Geometry check sheet. Reference: the model listing, model coordinates, mm. Face numbers are marked on the shaded views. A direction names the side the tool comes from. Round coordinates to 2 decimals unless told otherwise and drop trailing zeros.
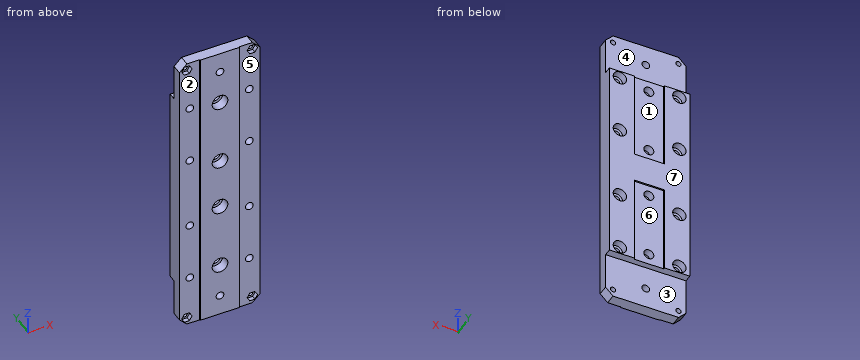
```python
from build123d import *

# Parameters (mm, degrees)
SKETCH1_W               = 54
SKETCH1_H               = 200
SKETCH1_R               = 2.6
SKETCH1_R_2             = 3.35
BOSS_EXTRUDE1_DEPTH     = 12
SKETCH4_R               = 5.25
CUT_EXTRUDE2_DEPTH      = 6
CUT_EXTRUDE3_START      = 12
SKETCH5_W               = 20
SKETCH5_H               = 60
CUT_EXTRUDE3_DEPTH      = 1
CUT_EXTRUDE4_DEPTH      = 105.273678366
CUT_EXTRUDE4_DEPTH_BACK = 105.273678366
SKETCH6_R               = 1.75
CUT_EXTRUDE5_DEPTH      = 3
CHAMFER2_SIZE           = 5
BOSS_EXTRUDE3_START     = -0.5
SKETCH9_W               = 27
SKETCH9_H               = 200
SKETCH9_R               = 2.6
SKETCH9_R_2             = 5.25
BOSS_EXTRUDE3_DEPTH     = 0.5
CHAMFER3_SIZE           = 0.5
SKETCH10_W              = 54
SKETCH10_H              = 30
CUT_EXTRUDE6_DEPTH      = 5
CUT_EXTRUDE7_START      = 12
SKETCH11_R              = 4.5
CUT_EXTRUDE7_DEPTH      = 5


with BuildPart() as part:
    # Sketch1 → Boss-Extrude1 (new body)
    with BuildSketch(Plane(origin=(0, 0, 0), x_dir=(1, 0, 0), z_dir=(0, 1, 0))):
        Rectangle(SKETCH1_W, SKETCH1_H)
        with Locations(Location((0, 86, 0), (0, 0, 270))):
            Circle(SKETCH1_R, mode=Mode.SUBTRACT)
        with Locations(Location((0, -86, 0), (0, 0, 270))):
            Circle(SKETCH1_R, mode=Mode.SUBTRACT)
        with Locations(Location((0, 62.5, 0), (0, 0, 270))):
            Circle(SKETCH1_R_2, mode=Mode.SUBTRACT)
        with Locations(Location((0, 17.5, 0), (0, 0, 270))):
            Circle(SKETCH1_R_2, mode=Mode.SUBTRACT)
        with Locations(Location((0, -17.5, 0), (0, 0, 270))):
            Circle(SKETCH1_R_2, mode=Mode.SUBTRACT)
        with Locations(Location((0, -62.5, 0), (0, 0, 270))):
            Circle(SKETCH1_R_2, mode=Mode.SUBTRACT)
        with Locations(Location((-20, -65, 0), (0, 0, 270))):
            Circle(SKETCH1_R, mode=Mode.SUBTRACT)
        with Locations(Location((20, -65, 0), (0, 0, 270))):
            Circle(SKETCH1_R, mode=Mode.SUBTRACT)
        with Locations(Location((20, -25, 0), (0, 0, 270))):
            Circle(SKETCH1_R, mode=Mode.SUBTRACT)
        with Locations(Location((-20, -25, 0), (0, 0, 270))):
            Circle(SKETCH1_R, mode=Mode.SUBTRACT)
        with Locations(Location((-20, 25, 0), (0, 0, 270))):
            Circle(SKETCH1_R, mode=Mode.SUBTRACT)
        with Locations(Location((20, 25, 0), (0, 0, 270))):
            Circle(SKETCH1_R, mode=Mode.SUBTRACT)
        with Locations(Location((20, 65, 0), (0, 0, 270))):
            Circle(SKETCH1_R, mode=Mode.SUBTRACT)
        with Locations(Location((-20, 65, 0), (0, 0, 270))):
            Circle(SKETCH1_R, mode=Mode.SUBTRACT)
    extrude(amount=BOSS_EXTRUDE1_DEPTH)

    # Sketch4 → Cut-Extrude2 (cut)
    with BuildSketch(Plane(origin=(0, 0, 0), x_dir=(1, 0, 0), z_dir=(0, 1, 0))):
        with Locations(Location((0, 62.5, 0), (0, 0, 270))):
            Circle(SKETCH4_R)
        with Locations(Location((0, 17.5, 0), (0, 0, 270))):
            Circle(SKETCH4_R)
        with Locations(Location((0, -17.5, 0), (0, 0, 270))):
            Circle(SKETCH4_R)
        with Locations(Location((0, -62.5, 0), (0, 0, 270))):
            Circle(SKETCH4_R)
    extrude(amount=CUT_EXTRUDE2_DEPTH, mode=Mode.SUBTRACT)

    # Sketch5 → Cut-Extrude3 (cut)
    with BuildSketch(Plane(origin=(0, 0, 0), x_dir=(1, 0, 0), z_dir=(0, 1, 0)).offset(CUT_EXTRUDE3_START)):
        with Locations((0, 40)):
            Rectangle(SKETCH5_W, SKETCH5_H)
        with Locations((0, -40)):
            Rectangle(SKETCH5_W, SKETCH5_H)
    extrude(amount=-CUT_EXTRUDE3_DEPTH, mode=Mode.SUBTRACT)

    # Sketch6 → Cut-Extrude4 (cut, two sides: drawn at the far end of the back side and taken through both)
    with BuildSketch(Plane(origin=(0, 0, 0), x_dir=(1, 0, 0), z_dir=(0, 1, 0)).offset(-CUT_EXTRUDE4_DEPTH_BACK)):
        with Locations(Location((22, 95, 0), (0, 0, 90))):
            Circle(SKETCH6_R)
        with Locations(Location((22, -95, 0), (0, 0, 90))):
            Circle(SKETCH6_R)
        with Locations(Location((-22, -95, 0), (0, 0, 90))):
            Circle(SKETCH6_R)
        with Locations(Location((-22, 95, 0), (0, 0, 90))):
            Circle(SKETCH6_R)
    extrude(amount=CUT_EXTRUDE4_DEPTH + CUT_EXTRUDE4_DEPTH_BACK, mode=Mode.SUBTRACT)

    # Sketch7 → Cut-Extrude5 (cut)
    with BuildSketch(Plane(origin=(0, 0, 0), x_dir=(1, 0, 0), z_dir=(0, 1, 0))):
        Polygon((18.535898385, 95), (20.267949192, 92), (23.732050808, 92), (25.464101615, 95), (23.732050808, 98), (20.267949192, 98), align=None)
        Polygon((18.535898385, -95), (20.267949192, -98), (23.732050808, -98), (25.464101615, -95), (23.732050808, -92), (20.267949192, -92), align=None)
        Polygon((-25.464101615, -95), (-23.732050808, -98), (-20.267949192, -98), (-18.535898385, -95), (-20.267949192, -92), (-23.732050808, -92), align=None)
        Polygon((-25.464101615, 95), (-23.732050808, 92), (-20.267949192, 92), (-18.535898385, 95), (-20.267949192, 98), (-23.732050808, 98), align=None)
    extrude(amount=CUT_EXTRUDE5_DEPTH, mode=Mode.SUBTRACT)

    # Chamfer2
    chamfer2_edges = [part.edges().sort_by_distance(p)[0] for p in [
        (27, 6, 100),
        (-27, 6, 100),
        (-27, 6, -100),
        (27, 6, -100),
    ]]
    chamfer(chamfer2_edges, length=CHAMFER2_SIZE)

    # Sketch9 → Boss-Extrude3 (add)
    with BuildSketch(Plane(origin=(0, 0, 0), x_dir=(1, 0, 0), z_dir=(0, 1, 0)).offset(BOSS_EXTRUDE3_START)):
        Rectangle(SKETCH9_W, SKETCH9_H)
        with Locations(Location((0, -86, 0), (0, 0, 270))):
            Circle(SKETCH9_R, mode=Mode.SUBTRACT)
        with Locations(Location((0, -62.5, 0), (0, 0, 270))):
            Circle(SKETCH9_R_2, mode=Mode.SUBTRACT)
        with Locations(Location((0, -17.5, 0), (0, 0, 270))):
            Circle(SKETCH9_R_2, mode=Mode.SUBTRACT)
        with Locations(Location((0, 17.5, 0), (0, 0, 270))):
            Circle(SKETCH9_R_2, mode=Mode.SUBTRACT)
        with Locations(Location((0, 62.5, 0), (0, 0, 270))):
            Circle(SKETCH9_R_2, mode=Mode.SUBTRACT)
        with Locations(Location((0, 86, 0), (0, 0, 270))):
            Circle(SKETCH9_R, mode=Mode.SUBTRACT)
    extrude(amount=BOSS_EXTRUDE3_DEPTH)

    # Chamfer3
    chamfer3_edges = [part.edges().sort_by_distance(p)[0] for p in [
        (-13.5, -0.5, 0),
        (13.5, -0.5, 0),
    ]]
    chamfer(chamfer3_edges, length=CHAMFER3_SIZE - 0.0001)  # a hair under: the kernel refuses the full size

    # Sketch10 → Cut-Extrude6 (cut)
    with BuildSketch(Plane(origin=(0, 12, 0), x_dir=(1, 0, 0), z_dir=(0, 1, 0))):
        with Locations((0, -85)):
            Rectangle(SKETCH10_W, SKETCH10_H)
        with Locations((0, 85)):
            Rectangle(SKETCH10_W, SKETCH10_H)
    extrude(amount=-CUT_EXTRUDE6_DEPTH, mode=Mode.SUBTRACT)

    # Sketch11 → Cut-Extrude7 (cut)
    with BuildSketch(Plane(origin=(0, 0, 0), x_dir=(1, 0, 0), z_dir=(0, 1, 0)).offset(CUT_EXTRUDE7_START)):
        with Locations(Location((20, 65, 0), (0, 0, 90))):
            Circle(SKETCH11_R)
        with Locations(Location((-20, 65, 0), (0, 0, 90))):
            Circle(SKETCH11_R)
        with Locations(Location((-20, 25, 0), (0, 0, 90))):
            Circle(SKETCH11_R)
        with Locations(Location((20, 25, 0), (0, 0, 90))):
            Circle(SKETCH11_R)
        with Locations(Location((20, -25, 0), (0, 0, 90))):
            Circle(SKETCH11_R)
        with Locations(Location((-20, -25, 0), (0, 0, 90))):
            Circle(SKETCH11_R)
        with Locations(Location((-20, -65, 0), (0, 0, 90))):
            Circle(SKETCH11_R)
        with Locations(Location((20, -65, 0), (0, 0, 90))):
            Circle(SKETCH11_R)
    extrude(amount=-CUT_EXTRUDE7_DEPTH, mode=Mode.SUBTRACT)


solid = part.part
```
1) Gauge pin test, flat ends, axial feed: pin 1 (4.5 mm diameter, centred on x = 22, z = 95, fed in from -Y); pin 2 (4 mm diameter, centred on x = -20, z = 65, fed in from +Y); pin 3 (1.5 mm diameter, centred on x = 5.5, y = 8.5, fed in from +Z); pin 4 (7 mm diameter, centred on x = -19, z = 24, fed in from +Y). Record the tip position at first contact, or that the pin passes through.
Report:
pin 1: stops at y = 3
pin 2: passes through
pin 3: stops at z = 70
pin 4: stops at y = 12
2) Sectioned sample at B-B, the plane z = 25. State how many separate pieces and enclosed holes the cut face has, then the cut area to 3 significant figures.
Report:
separate pieces: 3
enclosed holes: 0
area: 478 mm2
3) Mould release check, pull along X, two halves, no side actions. Record for the marked faces 1 and 2: +X half, -X half, draft (parallel to the pull), parting line (faces both ways), or undercut.
Report:
face 1: undercut
face 2: draft
4) Access from +Z, -Z, +X, -X, +Y, -Y to the whole of each face (thin tool, end or side, straight path). Record for the marked faces 3, 4, 5, 6 and 7.
Report:
face 3: -Z, +X, -X, +Y
face 4: +Z, +X, -X, +Y
face 5: +Z, -Z, +X, -Y
face 6: -Z, +Y
face 7: +Z, -Z, +X, -X, +Y
5) Scan lines: line 1 along Z through (x, y) = (0, 9); line 2 along X through (y, z) = (9.3, -25); line 3 along Z through (x, y) = (20, 5.75). Record each from-to range of solid material in increasing order.
Report:
line 1: z = -70 to -65.85, -59.15 to -20.85, -14.15 to 14.15, 20.85 to 59.15, 65.85 to 70
line 2: x = -27 to -24.5, -15.5 to 15.5, 24.5 to 27
line 3: z = -100 to -67.6, -62.4 to -27.6, -22.4 to 22.4, 27.6 to 62.4, 67.6 to 100
